Can you work these out from the model? Positions are in its coordinate system, mm. A direction names the side the tool comes from. Round coordinates to 2 decimals unless told otherwise and drop trailing zeros. Loops run counter-clockwise (first coordinate to the right, second up) from the corner with the lowest first, then second, coordinate; pieces in that order, holes last.
(1) If I drill on line 1 along Y through (x, z) = (0, 2.1); line 2 along Y through (x, z) = (0, 7.5); line 3 along Z through (x, y) = (4, -7), over which ranges is the centre line in solid material (lowest first)?
(2) I want a section at C-C on z = 8.75. Write out the boundary of the cut face in (x, y).
(3) Which directions (+Z, -Z, +X, -X, +Y, -Y) give clear straight access to the entire face, cutting with the end or side of a thin tool? Please do faces 1 (the face through (-1.172, 8.923, 13.028)), 2 (the face through (-8.3, 4.3, 0)), 3 (the face through (-1.172, 8.923, 1.972)).
(4) Thinking about a two-plate mould opening in Y: for faces 4 (the face through (-8.3, 4.3, 15)), 5 (the face through (-2.343, 17.847, 7.395)), 6 (the face through (0, -4, 11)), which applies, released by +Y, released by -Y, zero draft, split by the parting line, or undercut?
(5) I want a section at D-D on x = -5.5. Write out the boundary of the cut face in (y, z).
(6) I want a section at A-A on y = 0. Write out the boundary of the cut face in (x, z).
(7) Will these pins go through, and if not, where does the flat tip stop? pin 1 Ø6 at (x, z) = (-11, 8.5) entering from +Y; pin 2 Ø10.5 at (x, y) = (0, 0) entering from +Z; pin 3 Ø5 at (y, z) = (-12, 6) entering from -X.
from build123d import *

# Parameters (mm, degrees)
F0_R     = 18
F1_DEPTH = 15
F2_R     = 9
F2_R_2   = 3.25
F3_DEPTH = 4
F4_DEPTH = 25
F5_R     = 9
F6_DEPTH = 4


with BuildPart() as f1:
    # F0 (on Top) → F1 (new body)
    with BuildSketch(Plane.XY):
        Circle(F0_R)
    extrude(amount=F1_DEPTH)

    # F2 (on face) → F3 (cut)
    with BuildSketch(Plane.XY.offset(15)):
        Circle(F2_R)
        Circle(F2_R_2, mode=Mode.SUBTRACT)
    extrude(amount=-F3_DEPTH, mode=Mode.SUBTRACT)

    # F2 (on face) → F4 (cut)
    with BuildSketch(Plane.XY.offset(15)):
        Circle(F2_R_2)
    extrude(amount=-F4_DEPTH, mode=Mode.SUBTRACT)

    # F5 (on face) → F6 (cut)
    with BuildSketch(Plane.XY):
        Circle(F5_R)
    extrude(amount=F6_DEPTH, mode=Mode.SUBTRACT)


solid = f1.part
Filled sheet:
1. line 1: y = -18 to -9, 9 to 18
1. line 2: y = -18 to -3.25, 3.25 to 18
1. line 3: z = 4 to 11
2. outline: circle Ø36 at (0, 0); hole circle Ø6.5 at (0, 0)
3. face 1: +Z
3. face 2: -Z, +X, -X, +Y, -Y
3. face 3: -Z
4. face 4: zero draft
4. face 5: split by the parting line
4. face 6: undercut
5. outline: (-17.14, 0) - (-7.12, 0) - (-7.12, 4) - (7.12, 4) - (7.12, 0) - (17.14, 0) - (17.14, 15) - (7.12, 15) - (7.12, 11) - (-7.12, 11) - (-7.12, 15) - (-17.14, 15) - close
6. outline: (-18, 0) - (-9, 0) - (-9, 4) - (-3.25, 4) - (-3.25, 11) - (-9, 11) - (-9, 15) - (-18, 15) - close; (3.25, 4) - (9, 4) - (9, 0) - (18, 0) - (18, 15) - (9, 15) - (9, 11) - (3.25, 11) - close
7. pin 1: stops at y = 16.12
7. pin 2: stops at z = 11
7. pin 3: stops at x = -15.29
